Geometry check sheet. Reference: the model listing, model coordinates, mm. Round coordinates to 2 decimals unless told otherwise and drop trailing zeros. Order: outer loops, then holes, each group sorted by start corner. A loop starts at its lowest first (then second) coordinate and runs counter-clockwise, first axis right, second up.
(1) Cross-section at D-D on y = 34. Enter the section's corners in (x, z), and give its area (3 significant figures).
(2) Cross-section at C-C on z = 1.95. Count the separate pieces of the cut face and the enclosed holes in it, and give its area (3 significant figures).
(3) Cross-section at A-A on y = 0. Enter the section's corners in (x, z), and give its area (3 significant figures).
(4) Thickness scan on L1, parallel to X at y = -0.5, z = 2.2; L2, parallel to Y at x = -27.5, z = 2.3; L3, parallel to Y at x = -22.5, z = 2. Record the ranges inside material, lowest first.
(5) Cross-section at B-B on x = 0. Enter the section's corners in (y, z).
(6) Gauge pin test, flat ends, axial feed: P1, Ø2.5, axis at x = 23.53, y = -23.53, coming from the +Z side; P2, Ø5, axis at x = -50.65, y = -50.65, coming from the +Z side; P3, Ø1.3, axis at x = -6, z = 1, coming from the -Y side; P4, Ø1.3, axis at y = -1, z = 0.5, coming from the +X side. Record the tip position at first contact, or that the pin passes through.
from build123d import *

# Parameters (mm, degrees)
SKETCH1_R           = 76.2
SKETCH1_R_2         = 2.54
SKETCH1_R_3         = 1.905
SKETCH1_W           = 39.878
SKETCH1_H           = 19.939
BOSS_EXTRUDE1_DEPTH = 2.54


with BuildPart() as part:
    # Sketch1 → Boss-Extrude1 (new body)
    with BuildSketch(Plane.XY):
        Circle(SKETCH1_R)
        with Locations((14.732, -4.8895)):
            Circle(SKETCH1_R_2, mode=Mode.SUBTRACT)
        with Locations((14.732, 4.8895)):
            Circle(SKETCH1_R_2, mode=Mode.SUBTRACT)
        with Locations((-35.814, 4.8895)):
            Circle(SKETCH1_R_2, mode=Mode.SUBTRACT)
        with Locations((-35.814, -4.8895)):
            Circle(SKETCH1_R_2, mode=Mode.SUBTRACT)
        with Locations((23.528271037, 23.528271037)):
            Circle(SKETCH1_R_3, mode=Mode.SUBTRACT)
        with Locations((23.528271037, -23.528271037)):
            Circle(SKETCH1_R_3, mode=Mode.SUBTRACT)
        with Locations((-23.528271037, -23.528271037)):
            Circle(SKETCH1_R_3, mode=Mode.SUBTRACT)
        with Locations((-23.528271037, 23.528271037)):
            Circle(SKETCH1_R_3, mode=Mode.SUBTRACT)
        with Locations((50.648644523, 50.648644523)):
            Circle(SKETCH1_R_3, mode=Mode.SUBTRACT)
        with Locations((50.648644523, -50.648644523)):
            Circle(SKETCH1_R_3, mode=Mode.SUBTRACT)
        with Locations((-50.648644523, -50.648644523)):
            Circle(SKETCH1_R_3, mode=Mode.SUBTRACT)
        with Locations((-50.648644523, 50.648644523)):
            Circle(SKETCH1_R_3, mode=Mode.SUBTRACT)
        with Locations((-10.541, 0)):
            Rectangle(SKETCH1_W, SKETCH1_H, mode=Mode.SUBTRACT)
        with BuildLine():
            Line((-44.901280605, -44.901280605), (-31.430896424, -31.430896424))
            ThreePointArc((-31.430896424, -31.430896424), (0, -44.45), (31.430896424, -31.430896424))
            Line((31.430896424, -31.430896424), (44.901280605, -44.901280605))
            ThreePointArc((44.901280605, -44.901280605), (0, -63.5), (-44.901280605, -44.901280605))
        make_face(mode=Mode.SUBTRACT)
        with BuildLine():
            Line((44.901280605, 44.901280605), (31.430896424, 31.430896424))
            ThreePointArc((31.430896424, 31.430896424), (0, 44.45), (-31.430896424, 31.430896424))
            Line((-31.430896424, 31.430896424), (-44.901280605, 44.901280605))
            ThreePointArc((-44.901280605, 44.901280605), (0, 63.5), (44.901280605, 44.901280605))
        make_face(mode=Mode.SUBTRACT)
    extrude(amount=BOSS_EXTRUDE1_DEPTH)


solid = part.part
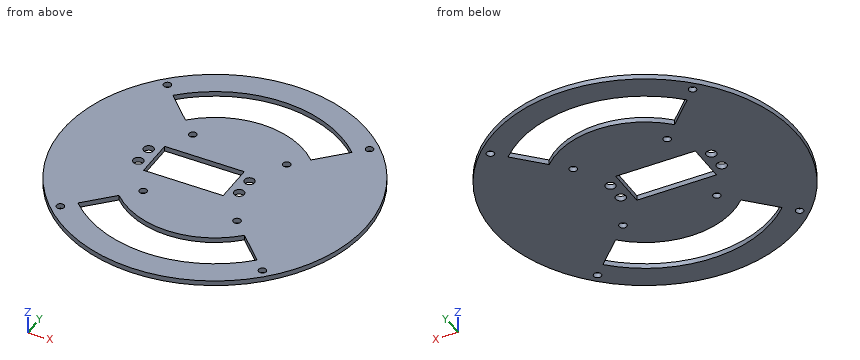
Found:
1. outline: (-68.19, 0) - (-34, 0) - (-34, 2.54) - (-68.19, 2.54) - close; (-28.63, 0) - (28.63, 0) - (28.63, 2.54) - (-28.63, 2.54) - close; (34, 0) - (68.19, 0) - (68.19, 2.54) - (34, 2.54) - close
1. area: 319 mm2
2. separate pieces: 1
2. enclosed holes: 15
2. area: 14,000 mm2
3. outline: (-76.2, 0) - (-30.48, 0) - (-30.48, 2.54) - (-76.2, 2.54) - close; (9.4, 0) - (76.2, 0) - (76.2, 2.54) - (9.4, 2.54) - close
3. area: 286 mm2
4. L1: x = -76.2 to -30.48, 9.4 to 76.2
4. L2: y = -71.06 to -57.24, -34.92 to -9.97, 9.97 to 34.92, 57.24 to 71.06
4. L3: y = -72.8 to -59.38, -38.33 to -25.13, -21.92 to -9.97, 9.97 to 21.92, 25.13 to 38.33, 59.38 to 72.8
5. outline: (-76.2, 0) - (-63.5, 0) - (-63.5, 2.54) - (-76.2, 2.54) - close; (-44.45, 0) - (-9.97, 0) - (-9.97, 2.54) - (-44.45, 2.54) - close; (9.97, 0) - (44.45, 0) - (44.45, 2.54) - (9.97, 2.54) - close; (63.5, 0) - (76.2, 0) - (76.2, 2.54) - (63.5, 2.54) - close
6. P1: passes through
6. P2: stops at z = 2.54
6. P3: stops at y = -76.01
6. P4: stops at x = 76.2
